Build history of the part. All positions in model axes, mm. Round coordinates to 2 decimals unless told otherwise and drop trailing zeros. Write each loop counter-clockwise with the first axis right and the second up, starting at its lowest first coordinate (ties: lowest second). Pieces come first, ordered by that corner, then holes. Notation, with made-up numbers: (-9.5, 14.25) -> (28.5, 14.25) arc R14 ccw to (28.5, 18.25) -> close; hole circle Ø10 at (-38.75, 53). An arc over 180 degrees is marked (long way). Answer in a Markdown table with one row per item. Add a question column.
from build123d import *

# Parameters (mm, degrees)
F1_DEPTH = 6
F2_R     = 1
F3_DEPTH = 110


with BuildPart() as f1:
    # F0 (on Front) → F1 (new body)
    with BuildSketch(Plane.XZ):
        Polygon((-31.122757, 104), (-31.122757, 0), (48.877243, 0), (48.877243, 96), align=None)
    extrude(amount=F1_DEPTH)

    # F2 (on Top) → F3 (cut)
    with BuildSketch(Plane.XY):
        with Locations((-21.149542, -3)):
            Circle(F2_R)
        with Locations((-11.149542, -3)):
            Circle(F2_R)
        with Locations((-1.149542, -3)):
            Circle(F2_R)
        with Locations((8.850458, -3)):
            Circle(F2_R)
        with Locations((18.850458, -3)):
            Circle(F2_R)
        with Locations((28.850458, -3)):
            Circle(F2_R)
        with Locations((38.850458, -3)):
            Circle(F2_R)
    extrude(amount=F3_DEPTH, mode=Mode.SUBTRACT)


solid = f1.part
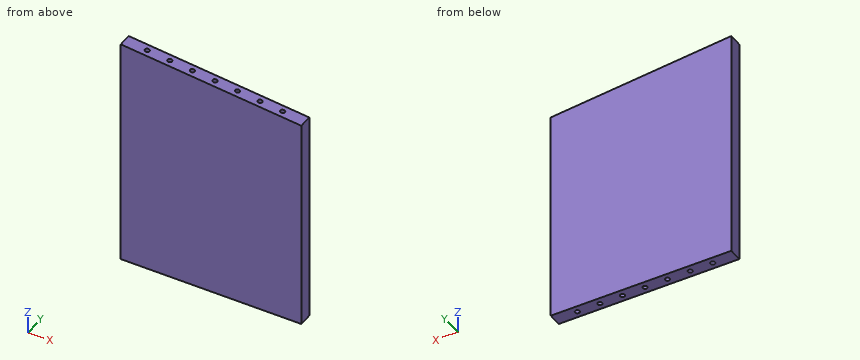
(1) Saw through at A-A (z = 62). List the corners of the cut face in (x, y), plus the area to 3 significant figures.
(2) Probe line 1 along Y through (x, z) = (-11, 24.5); line 2 along Y through (x, z) = (-1.5, 89.5); line 3 along Z through (x, y) = (28.5, -5.4). List the from-to ranges inside material, lowest first.
(3) Saw through at C-C (x = -7). List the corners of the cut face in (y, z).
(4) Drop flat-ended pins along their axis: P1, Ø2.5, axis at x = -11.15, y = -3, coming from the +Z side; P2, Ø2, axis at x = -4, y = -4.5, coming from the +Z side. Give the stop position or say it passes through.
(5) Saw through at D-D (x = 35). List the corners of the cut face in (y, z).
(6) Saw through at B-B (y = -3). Count the separate pieces of the cut face and the enclosed holes in it, plus the area to 3 significant figures.
Answer sheet:
| question | item | result |
|---|---|---|
| 1 | outline | (-31.12, -6) -> (48.88, -6) -> (48.88, 0) -> (-31.12, 0) -> close; hole circle Ø2 at (-21.15, -3); hole circle Ø2 at (-11.15, -3); hole circle Ø2 at (-1.15, -3); hole circle Ø2 at (8.85, -3); hole circle Ø2 at (18.85, -3); hole circle Ø2 at (28.85, -3); hole circle Ø2 at (38.85, -3) |
| 1 | area | 458 mm² |
| 2 | line 1 | y = -6 to -3.99, -2.01 to 0 |
| 2 | line 2 | y = -6 to -3.94, -2.06 to 0 |
| 2 | line 3 | z = 0 to 98.04 |
| 3 | outline | (-6, 0) -> (0, 0) -> (0, 101.59) -> (-6, 101.59) -> close |
| 4 | P1 | stops at z = 102.13 |
| 4 | P2 | stops at z = 101.39 |
| 5 | outline | (-6, 0) -> (0, 0) -> (0, 97.39) -> (-6, 97.39) -> close |
| 6 | separate pieces | 8 |
| 6 | enclosed holes | 0 |
| 6 | area | 6,600 mm² |
